Answer from the drawing. Dimensions are ordinates in mm from the lowest x, y and z of the part. Round coordinates to 2 decimals unless told otherwise and drop trailing zeros. Loops run counter-clockwise (first coordinate to the right, second up) from the corner with the lowest first, then second, coordinate; pieces in that order, holes last. Notation, with made-up numbers: M -34,-16 L -17,-16 A17 cw -17,17 Z; hole C 68,10 d8. An arc over 180 degrees is marked long. Answer as a JSON object with one key per item and string values.
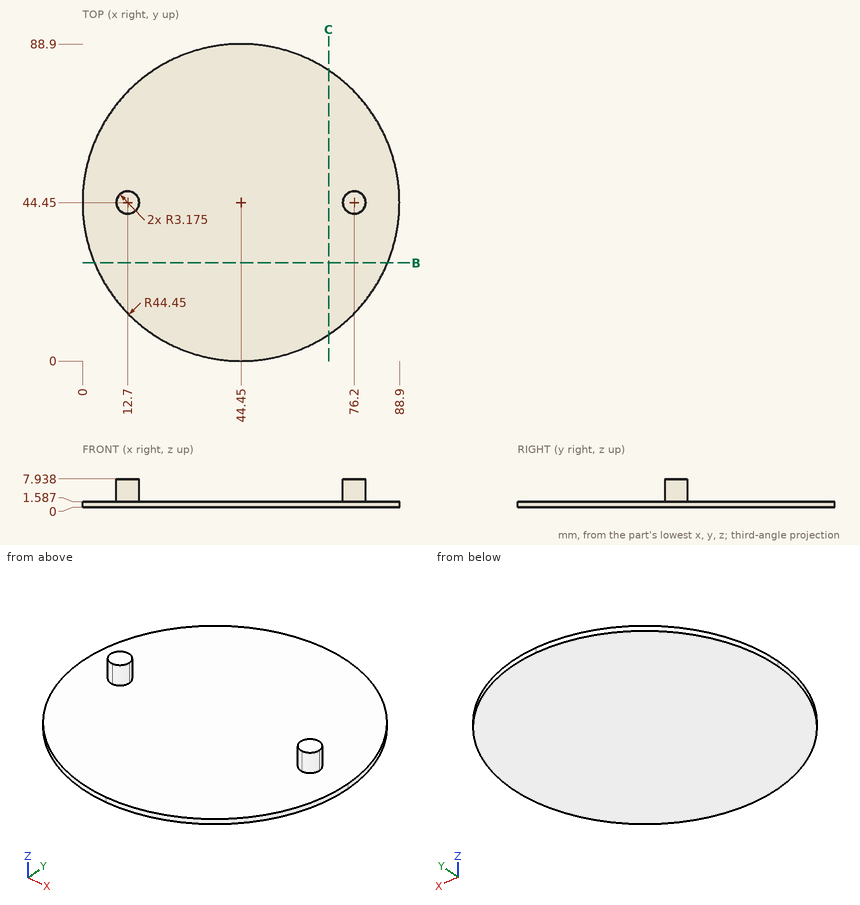
Item 1: The part is cut by section B-B (y = 27.5). Give the vertices of the cut face in (x, z).
Values follow:
{"outline": "M 3.36,0 L 85.54,0 L 85.54,1.59 L 3.36,1.59 Z"}
Item 2: Straight lines are drawn through the part: line 1 (Z direction, x = 29.5, y = 37.5); line 2 (Y direction, x = 13, z = 2.75); line 3 (X direction, y = 79, z = 1.5) (1 decimal). For each, find the intervals that lie inside material, in ascending order.
Values follow:
{"line 1": "0 to 1.59", "line 2": "41.29 to 47.61", "line 3": "16.5 to 72.4"}
Item 3: The part is cut by section C-C (x = 69). Give the vertices of the cut face in (y, z) (1 decimal).
Values follow:
{"outline": "M 7.4,0 L 81.5,0 L 81.5,1.6 L 7.4,1.6 Z"}
Item 4: Flat-ended cylindrical pins translate along their axes: P1, Ø1.5, axis at x = 37.5, y = 67.5, coming from the +Z side; P2, Ø2, axis at y = 47.5, z = 3, coming from the +X side (1 decimal). Find the tip coordinate at first contact, or state that the pin passes through.
Values follow:
{"P1": "z = 1.59", "P2": "x = 78.6"}
